Autodesk Inventor part; units mm, degrees
ref_plane "YZ Plane" through (0, 0, 0) normal (1, 0, 0) x (0, 1, 0)
ref_plane "XZ Plane" through (0, 0, 0) normal (0, 1, 0) x (-1, 0, 0)
ref_plane "XY Plane" through (0, 0, 0) normal (0, 0, 1) x (1, 0, 0)
sketch "Sketch1" plane through (0, 0, 0) normal (1, 0, 0) x (0, 1, 0)
  line L0 (12.0042, 143.7964) -> (-27.9958, 143.7964)
  line L1 (-27.9958, 143.7964) -> (-27.9958, -156.2036)
  line L2 (-27.9958, -156.2036) -> (12.0042, -156.2036)
  line L3 (12.0042, -156.2036) -> (12.0042, 143.7964)
  point P0 (0, 0)
  dimension "d0" = 300
  dimension "d1" = 40
extrude "Extrusion1" add sketch "Sketch1" along normal blind 30
sketch "Sketch2" plane through (30, 0, 0) normal (1, 0, 0) x (0, 0, -1)
  circle A0 centre (-123.621, -6.7738) radius 12.1593
  circle A1 centre (130.9593, -6.7738) radius 13.5475
  point P0 (0, 0)
extrude "Extrusion2" cut sketch "Sketch2" against normal blind 30
properties part number "ejemplo_tibia"
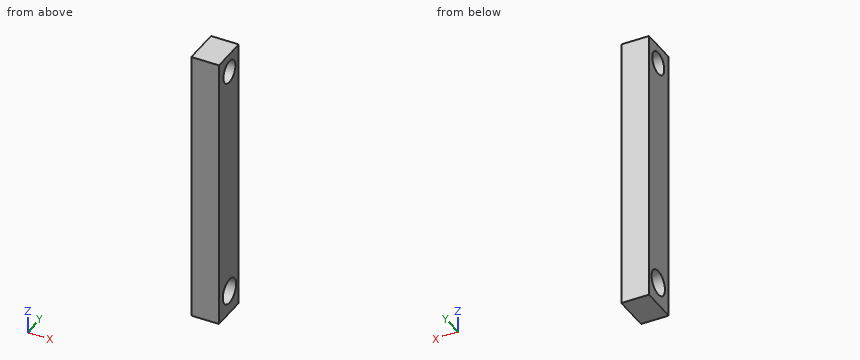
Can you work these out from the model? Positions are in its coordinate system, mm. Coordinates: 2 decimals unless noted, no trailing zeros. Loops run counter-clockwise (first coordinate to the right, second up) from the corner with the lowest first, then second, coordinate; pieces in that order, holes last. Notation, with made-up numbers: M 50.25,-27.75 L 67.25,-27.75 A23 ccw 67.25,3.25 Z; hole C -11,15 d10. An arc over 180 degrees is marked long. Return JSON: item names as keys, results as strings. Group by question number.
Item 1: If I drill on L1, parallel to Z at x = 17, y = -1.5; L2, parallel to Z at x = 23.25, y = -5; L3, parallel to Z at x = 21.75, y = -19, over which ranges is the centre line in solid material (lowest first)? Write a range as from..to.
Item 2: Imagine slicing it at B-B (z = 114). Please give me the cut outline in (x, y), and give its area (3 significant figures).
Item 3: Imagine slicing it at A-A (y = -0.5). Please give me the cut outline in (x, z).
Item 4: Imagine slicing it at D-D (x = 13.75). Please give me the cut outline in (y, z) (1 decimal).
Item 5: Imagine slicing it at C-C (y = -16). Please give me the cut outline in (x, z).
Verdict:
{
 "1": {"L1": "z = -156.2..-143.44, -118.48..112.66, 134.58..143.8", "L2": "z = -156.2..-144.39, -117.53..111.59, 135.65..143.8", "L3": "z = -156.2..-136.79, -125.12..143.8"},
 "2": {"outline": "M 0,-28 L 30,-28 L 30,-14.21 L 0,-14.21 Z; M 0,0.66 L 30,0.66 L 30,12 L 0,12 Z", "area": "754 mm^2"},
 "3": {"outline": "M 0,-156.2 L 30,-156.2 L 30,-142.97 L 0,-142.97 Z; M 0,-118.95 L 30,-118.95 L 30,113.21 L 0,113.21 Z; M 0,134.04 L 30,134.04 L 30,143.8 L 0,143.8 Z"},
 "4": {"outline": "M -28,-156.2 L 12,-156.2 L 12,143.8 L -28,143.8 Z; hole C -6.8,-131 d27.1; hole C -6.8,123.6 d24.3"},
 "5": {"outline": "M 0,-156.2 L 30,-156.2 L 30,-140.88 L 0,-140.88 Z; M 0,-121.04 L 30,-121.04 L 30,115.7 L 0,115.7 Z; M 0,131.54 L 30,131.54 L 30,143.8 L 0,143.8 Z"}
}
